from build123d import *

# Parameters (mm, degrees)
SKETCH1_R           = 4.762499999999997
SKETCH1_R_2         = 3.17500000000001
SKETCH1_R_3         = 3.174999999999997
SKETCH1_R_4         = 4.000000000000006
BOSS_EXTRUDE1_DEPTH = 12.572999999999999
BOSS_EXTRUDE2_DEPTH = 0.889
SKETCH1_6_R         = 3.174999999999997
CUT_EXTRUDE1_DEPTH  = 6.477
SKETCH1_7_R         = 4.000000000000006
CUT_EXTRUDE2_DEPTH  = 8.889999999999999
CUT_EXTRUDE3_DEPTH  = 8.889999999999999
FILLET1_R           = 3.8099999999999996
FILLET2_R           = 3.175
FILLET3_R           = 12.7


with BuildPart() as part:
    # Sketch1 → Boss-Extrude1 (new, symmetric)
    with BuildSketch(Plane(origin=(0, 0, 0), x_dir=(0, 1, 0), z_dir=(0, 0, 1))):
        with BuildLine():
            ThreePointArc((20.382390084242772, 19.257386231100043), (20.978466310939545, 20.483226967362732), (21.356021010960387, 21.79297687753883))
            Line((21.356021010960387, 21.79297687753883), (37.358021010960385, 102.94546522066996))
            ThreePointArc((37.35802101096039, 102.94546522066996), (37.07094462485589, 107.07851604910101), (34.74047115882098, 110.5039233863327))
            Line((34.74047115882098, 110.5039233863327), (5.8316712608374885, 135.31904946315026))
            ThreePointArc((5.831671260837487, 135.31904946315026), (-1.9784012059195106, 136.6053065422467), (-6.71668575438994, 130.26493204642645))
            Line((-6.71668575438994, 130.26493204642645), (-14.21259444493871, 52.14693537573538))
            Line((-14.21259444493871, 52.14693537573538), (-7.56089550263359, -0.9472376672489283))
            ThreePointArc((-7.560895502633591, -0.9472376672489284), (-1.565846256947838, -7.457380605789306), (6.541359720008749, -3.9083261140093004))
            Line((6.541359720008749, -3.9083261140093004), (20.382390084242772, 19.257386231100043))
        make_face()
        with Locations(Location((3.33e-15, 1.67e-15, 0), (0, 0, 270))):
            Circle(SKETCH1_R, mode=Mode.SUBTRACT)
        Polygon((-1.3308119334704962, 9.509064286128918), (4.29827889322349, 19.45469368119458), (9.577469944104607, 16.46674342320252), (3.8313636145238874, 6.587343209590925), align=None, mode=Mode.SUBTRACT)
        with BuildLine():
            Line((-7.837469994075563, 15.563413639417114), (-10.493663341451699, 36.76527356188965))
            ThreePointArc((-10.493663341451697, 36.76527356188965), (-8.373880180823447, 40.66792915781828), (-3.9976174727208837, 39.91127464075849))
            Line((-3.9976174727208846, 39.91127464075849), (5.307057429865875, 30.45613112841883))
            ThreePointArc((5.307057429865875, 30.45613112841883), (6.368728770469758, 28.282081544681937), (5.907210919033615, 25.907078618197012))
            Line((5.907210919033615, 25.907078618197012), (-0.7412706361770095, 14.160362208064143))
            ThreePointArc((-0.7412706361770094, 14.160362208064143), (-4.796024243086445, 12.29938935959272), (-7.837469994075564, 15.563413639417115))
        make_face(mode=Mode.SUBTRACT)
        with Locations(Location((13.568473709233661, 23.328559266526405, 0), (0, 0, 270))):
            Circle(SKETCH1_R_2, mode=Mode.SUBTRACT)
        with BuildLine():
            Line((-9.835366262341573, 53.13228955360719), (15.923267523608242, 85.75989234914361))
            ThreePointArc((15.92326752360824, 85.75989234914361), (17.2521532494062, 86.82767112773601), (18.9136708602906, 87.20904760965752))
            Line((18.9136708602906, 87.20904760965752), (27.031501436121193, 87.20904760965755))
            ThreePointArc((27.031501436121193, 87.20904760965755), (29.974660714259272, 85.81853380790496), (30.769524140950022, 82.6619680629435))
            Line((30.769524140950015, 82.6619680629435), (21.11582108508837, 33.70421123824264))
            ThreePointArc((21.11582108508837, 33.70421123824264), (19.28061275870069, 31.140473092142116), (16.142341730197096, 30.837161643844155))
            ThreePointArc((16.142341730197096, 30.837161643844155), (13.427097985028178, 31.264800137027077), (10.728808005125181, 30.74072527511728))
            ThreePointArc((10.728808005125181, 30.74072527511728), (8.557460112178255, 30.57529521299933), (6.650170349739085, 31.62618271399653))
            Line((6.650170349739083, 31.62618271399653), (-9.560561043073251, 48.099062568876725))
            ThreePointArc((-9.56056104307325, 48.099062568876725), (-10.649296851393418, 50.56373496479325), (-9.835366262341573, 53.13228955360719))
        make_face(mode=Mode.SUBTRACT)
        with BuildLine():
            ThreePointArc((-6.271634521139667, 108.31101038198426), (-5.0412373021941335, 110.76689735834775), (-2.4790547893278805, 111.75708871754208))
            Line((-2.4790547893278805, 111.75708871754208), (11.028473709233646, 111.75708871754206))
            ThreePointArc((11.028473709233646, 111.75708871754206), (13.722550545554382, 110.6411655538628), (14.838473709233643, 107.94708871754207))
            Line((14.838473709233645, 107.94708871754207), (14.838473709233652, 89.90058630028007))
            ThreePointArc((14.83847370923365, 89.90058630028007), (14.417020328206092, 87.40152116017657), (13.199280382598367, 85.17889682130792))
            Line((13.199280382598367, 85.17889682130792), (-3.473328559543596, 64.06025882792814))
            ThreePointArc((-3.473328559543596, 64.06025882792814), (-7.883928971008091, 62.885691247927234), (-10.256311628037745, 66.7850252318564))
            Line((-10.256311628037743, 66.7850252318564), (-6.271634521139673, 108.31101038198426))
        make_face(mode=Mode.SUBTRACT)
        with Locations(Location((29.57047370923365, 104.48104760965752, 0), (0, 0, 270))):
            Circle(SKETCH1_R_3, mode=Mode.SUBTRACT)
        with Locations(Location((0.868473709233646, 129.5370887175421, 0), (0, 0, 270))):
            Circle(SKETCH1_R_4, mode=Mode.SUBTRACT)
    extrude(amount=BOSS_EXTRUDE1_DEPTH, both=True)

    # Sketch1_5 → Boss-Extrude2 (add, symmetric)
    with BuildSketch(Plane(origin=(0, 0, 0), x_dir=(0, 1, 0), z_dir=(0, 0, 1))):
        with BuildLine():
            Line((11.028473709233646, 111.75708871754206), (-2.4790547893278805, 111.75708871754208))
            ThreePointArc((-2.4790547893278805, 111.75708871754208), (-5.0412373021941335, 110.76689735834775), (-6.271634521139667, 108.31101038198426))
            Line((-6.271634521139673, 108.31101038198426), (-10.256311628037743, 66.7850252318564))
            ThreePointArc((-10.256311628037745, 66.7850252318564), (-7.883928971008091, 62.885691247927234), (-3.473328559543596, 64.06025882792814))
            Line((-3.473328559543596, 64.06025882792814), (13.199280382598367, 85.17889682130792))
            ThreePointArc((13.199280382598367, 85.17889682130792), (14.417020328206092, 87.40152116017657), (14.83847370923365, 89.90058630028007))
            Line((14.838473709233652, 89.90058630028007), (14.838473709233645, 107.94708871754207))
            ThreePointArc((14.838473709233643, 107.94708871754207), (13.722550545554382, 110.6411655538628), (11.028473709233646, 111.75708871754206))
        make_face()
        with BuildLine():
            ThreePointArc((18.9136708602906, 87.20904760965752), (17.2521532494062, 86.82767112773601), (15.92326752360824, 85.75989234914361))
            Line((15.923267523608242, 85.75989234914361), (-9.835366262341573, 53.13228955360719))
            ThreePointArc((-9.835366262341573, 53.13228955360719), (-10.649296851393418, 50.56373496479325), (-9.56056104307325, 48.099062568876725))
            Line((-9.560561043073251, 48.099062568876725), (6.650170349739083, 31.62618271399653))
            ThreePointArc((6.650170349739085, 31.62618271399653), (8.557460112178255, 30.57529521299933), (10.728808005125181, 30.74072527511728))
            ThreePointArc((10.728808005125181, 30.74072527511728), (13.427097985028178, 31.264800137027077), (16.142341730197096, 30.837161643844155))
            ThreePointArc((16.142341730197096, 30.837161643844155), (19.28061275870069, 31.140473092142116), (21.11582108508837, 33.70421123824264))
            Line((21.11582108508837, 33.70421123824264), (30.769524140950015, 82.6619680629435))
            ThreePointArc((30.769524140950022, 82.6619680629435), (29.974660714259272, 85.81853380790496), (27.031501436121193, 87.20904760965755))
            Line((27.031501436121193, 87.20904760965755), (18.9136708602906, 87.20904760965752))
        make_face()
        with BuildLine():
            ThreePointArc((-3.9976174727208837, 39.91127464075849), (-8.373880180823447, 40.66792915781828), (-10.493663341451697, 36.76527356188965))
            Line((-10.493663341451699, 36.76527356188965), (-7.837469994075563, 15.563413639417114))
            ThreePointArc((-7.837469994075564, 15.563413639417115), (-4.796024243086445, 12.29938935959272), (-0.7412706361770094, 14.160362208064143))
            Line((-0.7412706361770095, 14.160362208064143), (5.907210919033615, 25.907078618197012))
            ThreePointArc((5.907210919033615, 25.907078618197012), (6.368728770469758, 28.282081544681937), (5.307057429865875, 30.45613112841883))
            Line((5.307057429865875, 30.45613112841883), (-3.9976174727208846, 39.91127464075849))
        make_face()
    extrude(amount=BOSS_EXTRUDE2_DEPTH, both=True)

    # Sketch1_6 → Cut-Extrude1 (cut, symmetric)
    with BuildSketch(Plane(origin=(0, 0, 0), x_dir=(0, 1, 0), z_dir=(0, 0, 1))):
        with BuildLine():
            Line((16.870473709233643, 89.24104760965754), (34.65572444447459, 89.24104760965754))
            Line((34.6557244444746, 89.24104760965753), (37.358021010960385, 102.94546522066996))
            ThreePointArc((37.35802101096039, 102.94546522066996), (37.07094462485589, 107.07851604910101), (34.74047115882098, 110.5039233863327))
            Line((34.74047115882098, 110.5039233863327), (16.870473709233643, 125.84341313577922))
            Line((16.870473709233647, 125.84341313577922), (16.870473709233643, 89.24104760965754))
        make_face()
        with Locations(Location((29.57047370923365, 104.48104760965752, 0), (0, 0, 270))):
            Circle(SKETCH1_6_R, mode=Mode.SUBTRACT)
    extrude(amount=CUT_EXTRUDE1_DEPTH, both=True, mode=Mode.SUBTRACT)

    # Sketch1_7 → Cut-Extrude2 (cut, symmetric)
    with BuildSketch(Plane(origin=(0, 0, 0), x_dir=(0, 1, 0), z_dir=(0, 0, 1))):
        with BuildLine():
            Line((14.838473709233647, 114.29708871754207), (14.838473709233648, 127.58766873843433))
            Line((14.83847370923364, 127.58766873843433), (5.831671260837486, 135.31904946315026))
            ThreePointArc((5.831671260837487, 135.31904946315026), (-1.9784012059195106, 136.6053065422467), (-6.71668575438994, 130.26493204642645))
            Line((-6.71668575438994, 130.26493204642645), (-8.248899849470712, 114.29708871754207))
            Line((-8.24889984947071, 114.29708871754207), (14.838473709233647, 114.29708871754207))
        make_face()
        with Locations(Location((0.868473709233646, 129.5370887175421, 0), (0, 0, 270))):
            Circle(SKETCH1_7_R, mode=Mode.SUBTRACT)
    extrude(amount=CUT_EXTRUDE2_DEPTH, both=True, mode=Mode.SUBTRACT)

    # Sketch1_9 → Cut-Extrude3 (cut, symmetric)
    with BuildSketch(Plane(origin=(0, 0, 0), x_dir=(0, 1, 0), z_dir=(0, 0, 1))):
        Polygon((10.542747734850291, 2.7887911737698072), (16.405901968121537, 12.601943867513532), (9.577469944104607, 16.46674342320252), (3.8313636145238874, 6.587343209590925), align=None)
    extrude(amount=CUT_EXTRUDE3_DEPTH, both=True, mode=Mode.SUBTRACT)

    # Fillet1
    fillet1_edges = [part.edges().sort_by_distance(p)[0] for p in [
        (-107.54223037271838, 16.870473709233643, 6.477),
        (-107.54223037271838, 16.870473709233643, -6.477),
        (-120.9423787279882, 14.838473709233647, -8.889999999999999),
        (-120.9423787279882, 14.838473709233647, 8.889999999999999),
        (-14.534343645358025, 12.99168595611307, 8.889999999999999),
        (-4.688067191680366, 7.1870556746870875, -8.889999999999999),
        (-14.534343645358025, 12.99168595611307, -8.889999999999999),
        (-4.688067191680366, 7.1870556746870875, 8.889999999999999),
    ]]
    fillet(fillet1_edges, radius=FILLET1_R)

    # Fillet2
    fillet2_edges = [part.edges().sort_by_distance(p)[0] for p in [
        (-89.24104760965754, 27.66809907685412, 6.477),
        (-89.24104760965754, 16.870473709233643, 0),
        (-89.24104760965754, 27.66809907685412, -6.477),
        (-89.24104760965754, 17.986396872912895, -5.3610768363207475),
        (-89.24104760965754, 17.986396872912895, 5.3610768363207475),
        (-114.29708871754207, 14.838473709233647, 0),
        (-114.29708871754207, 1.3897869298814687, 8.889999999999999),
        (-114.29708871754207, 1.3897869298814687, -8.889999999999999),
        (-114.29708871754207, 13.722550545554395, -7.774076836320745),
        (-114.29708871754207, 13.722550545554393, 7.774076836320746),
    ]]
    fillet(fillet2_edges, radius=FILLET2_R)

    # Fillet3
    fillet3_edges = [part.edges().sort_by_distance(p)[0] for p in [
        (-52.14693537573538, -14.21259444493871, 0),
    ]]
    fillet(fillet3_edges, radius=FILLET3_R)


solid = part.part
Could you check a few things on this model? Use its own coordinates, in mm. A direction names the side the tool comes from. Coordinates: 2 decimals unless noted, no trailing zeros. Loops run counter-clockwise (first coordinate to the right, second up) from the corner with the lowest first, then second, coordinate; pieces in that order, holes last.
1. For P1, Ø1.5, axis at x = -56.5, y = -1.5, coming from the -Z side; P2, Ø9, axis at y = 22, z = -6.5, coming from the +X side; P3, Ø8, axis at x = -120.5, z = -1.5, coming from the -Y side, each with a flat end and sliding along its axis, tell me the tip position at first contact or that it passes through.
2. For faces 1 (the face through (-39.747, -1.342, 6.813)), 2 (the face through (-122.771, 13.752, -7.744)), 3 (the face through (-5.58, 7.81, -7.74)), 4 (the face through (-2.364, 10.289, 0.176)), 5 (the face through (-20.12, 2.63, -6.65)), which set-ups out of +Z, -Z, +X, -X, +Y, -Y let a thin tool reach every point of the face, with its end or its side?
3. Imagine slicing it at A-A (x = -35). Please give me the cut outline in (y, z), and give its area (3 significant figures).
4. We'd pull the mould along Y, two halves only. Please class faces 6 (the face through (-122.771, 13.693, 7.804)), 7 (the face through (-125, 1, -8.89)), 8 (the face through (-58.53, 26.01, -6.81)), 9 (the face through (-104.89, 32.72, -9.57)): released by +Y, released by -Y, zero draft, split by the parting line, or undercut.
5. I need wall thicknesses on L1, parallel to Y at x = -67, z = 5.5; L2, parallel to Y at x = -23.5, z = -9.25; L3, parallel to X at y = 2, z = -6.5. Which ranges of each line are inside material? Lowest first, please.
6. Imagine slicing it at B-B (z = 11.25). Give the number of separate pieces and of enclosed holes in the cut face, and give its area (3 significant figures).
Computed values:
1. P1: stops at z = -0.89
1. P2: stops at x = -14.43
1. P3: stops at y = 14.69
2. face 1: +Z
2. face 2: -X, -Y
2. face 3: +Y
2. face 4: +Z, -Z, +X, +Y
2. face 5: -Z
3. outline: (-12.06, -12.57) - (-10.27, -12.57) - (-10.27, -0.89) - (0.84, -0.89) - (0.84, -12.57) - (3.33, -12.57) - (3.33, -0.89) - (21.37, -0.89) - (21.37, -12.57) - (23.96, -12.57) - (23.96, 12.57) - (21.37, 12.57) - (21.37, 0.89) - (3.33, 0.89) - (3.33, 12.57) - (0.84, 12.57) - (0.84, 0.89) - (-10.27, 0.89) - (-10.27, 12.57) - (-12.06, 12.57) - close
3. area: 225 mm2
4. face 6: released by -Y
4. face 7: zero draft
4. face 8: undercut
4. face 9: undercut
5. L1: y = -12.79 to -10.24, -1.15 to 1.11, 27.68 to 30.27
5. L2: y = -10.62 to -8.83, 4.54 to 10.4, 16.74 to 21.69
5. L3: x = -114.4 to -111.76, -70.99 to -68.12, -36.35 to -33.82, -19 to -15.39, -7.62 to -4.32, 4.32 to 7.35
6. separate pieces: 1
6. enclosed holes: 8
6. area: 2,160 mm2
